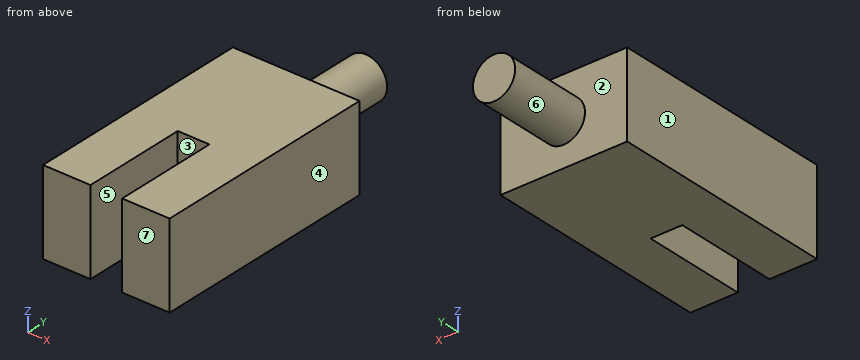
```python
from build123d import *

# Parameters (mm, degrees)
F1_DEPTH = 4
F2_R     = 1
F3_DEPTH = 4


with BuildPart() as f1:
    # F0 (on Top) → F1 (new body)
    with BuildSketch(Plane.XY):
        Polygon((-3.75, -32), (-3.75, -27), (-2.25, -27), (-2.25, -32), (0, -32), (0, -21.280894), (0, -21.118362), (-6, -21.118362), (-6, -32), align=None)
    extrude(amount=F1_DEPTH)

    # F2 (on face) → F3 (join)
    with BuildSketch(Plane(origin=(0, -21.118362, 0), x_dir=(-1, 0, 0), z_dir=(0, 1, 0))):
        with Locations((3, 2)):
            Circle(F2_R)
    extrude(amount=F3_DEPTH)


solid = f1.part
```
Can you work these out from the model? Positions are in its coordinate system, mm. Face numbers are marked on the shaded views. A direction names the side the tool comes from. Round coordinates to 2 decimals unless told otherwise and drop trailing zeros. Loops run counter-clockwise (first coordinate to the right, second up) from the corner with the lowest first, then second, coordinate; pieces in that order, holes last. Notation, with made-up numbers: (-31, 4) -> (-20, 4) arc R21 cw to (-20, 17) -> close; hole circle Ø4 at (-14, 57.5). An arc over 180 degrees is marked (long way). Answer in a Markdown table with one row per item.
Item 1: Suppose I cut it at C-C, the plane z = 2.8. List the corners of the cut face in (x, y) for me.
Answer block:
| item | result |
|---|---|
| outline | (-6, -32) -> (-3.75, -32) -> (-3.75, -27) -> (-2.25, -27) -> (-2.25, -32) -> (0, -32) -> (0, -21.12) -> (-2.4, -21.12) -> (-2.4, -17.12) -> (-3.6, -17.12) -> (-3.6, -21.12) -> (-6, -21.12) -> close |
Item 2: Suppose I cut it at D-D, the plane x = -1.8. List the corners of the cut face in (y, z) for me.
Answer block:
| item | result |
|---|---|
| outline | (-32, 0) -> (-21.12, 0) -> (-21.12, 4) -> (-32, 4) -> close |
Item 3: We'd pull the mould along X, two halves only. Please class the marked faces 1, 2, 3 and 4: released by +X, released by -X, zero draft, split by the parting line, or undercut.
Answer block:
| item | result |
|---|---|
| face 1 | released by -X |
| face 2 | zero draft |
| face 3 | undercut |
| face 4 | released by +X |
Item 4: Will this pin go through, and if not, where does the flat tip stop? P1, Ø0.8, axis at x = -3, z = 2, coming from the -Y side.
Answer block:
| item | result |
|---|---|
| P1 | y = -27 |
Item 5: On a 3-axis mill with a long thin cutter (end or side, diameter ignored), from which of +Z, -Z, +X, -X, +Y, -Y can I reach the whole of each face in a straight line? I mean the marked faces 5, 6 and 7. Say none if no direction works.
Answer block:
| item | result |
|---|---|
| face 5 | +Z, -Z, -Y |
| face 6 | +Y |
| face 7 | +Z, -Z, +X, -X, -Y |
Item 6: Suppose I cut it at B-B, the plane z = 2. List the corners of the cut face in (x, y) for me.
Answer block:
| item | result |
|---|---|
| outline | (-6, -32) -> (-3.75, -32) -> (-3.75, -27) -> (-2.25, -27) -> (-2.25, -32) -> (0, -32) -> (0, -21.12) -> (-2, -21.12) -> (-2, -17.12) -> (-4, -17.12) -> (-4, -21.12) -> (-6, -21.12) -> close |
Item 7: If I drill on probe 1 along X at (y, z) = (-28.5, 2.4); probe 2 along Y at (x, z) = (-2.15, 2.65); probe 3 along Y at (x, z) = (-3.3, 2.15), over which ranges is the centre line in solid material (lowest first)?
Answer block:
| item | result |
|---|---|
| probe 1 | -6 to -3.75, -2.25 to 0 |
| probe 2 | -32 to -21.12 |
| probe 3 | -27 to -17.12 |
Item 8: Suppose I cut it at A-A, the plane x = -3. List the corners of the cut face in (y, z) for me.
Answer block:
| item | result |
|---|---|
| outline | (-27, 0) -> (-21.12, 0) -> (-21.12, 1) -> (-17.12, 1) -> (-17.12, 3) -> (-21.12, 3) -> (-21.12, 4) -> (-27, 4) -> close |
